Model file for the job. Use its own axes, mm. Face numbers are marked on the shaded views. A direction names the side the tool comes from. Coordinates: 2 decimals unless noted, no trailing zeros. Loops run counter-clockwise (first coordinate to the right, second up) from the corner with the lowest first, then second, coordinate; pieces in that order, holes last.
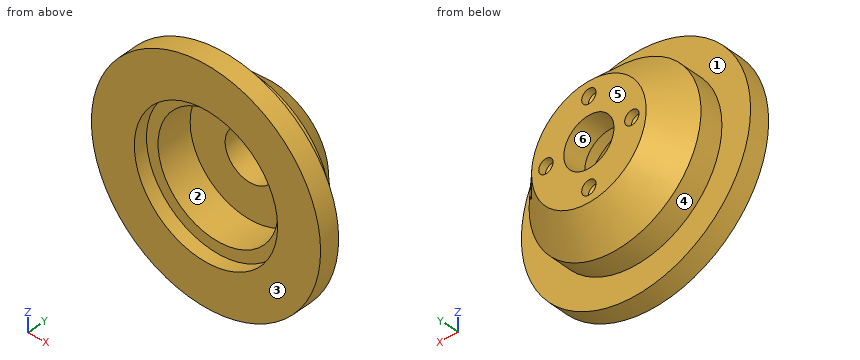
Autodesk Inventor part; units mm, degrees
ref_plane "Work Plane1" through (60, 0, 0) normal (1, 0, 0) x (0, 1, 0)
ref_plane "XZ Plane" through (0, 0, 0) normal (0, 1, 0) x (-1, 0, 0)
ref_plane "XY Plane" through (0, 0, 0) normal (0, 0, 1) x (1, 0, 0)
sketch "Sketch1" plane through (0, 0, 0) normal (0, 0, 1) x (1, 0, 0)
  line L0 (0, 0) -> (0, 66)
  line L1 (80, 0) -> (80, 13.8071)
  line L2 (-21.5975, 0) -> (0, 0)
  line L3 (46.9201, 0) -> (53.1744, 0)
  line L4 (80, 13.8071) -> (60, 13.8071)
  line L5 (60, 13.8071) -> (60, 33.8071)
  line L6 (36.9201, 33.8071) -> (30.3778, 33.8071)
  line L7 (0, 33.8071) -> (31.3863, 33.8071)
  line L8 (0, 33.8071) -> (0, 49.8071)
  line L9 (0, 49.8071) -> (35, 49.8071)
  line L10 (46.9201, 9.2823) -> (41.9201, 9.2823)
  line L11 (41.9201, 9.2823) -> (41.9201, 33.8071)
  line L12 (41.9201, 33.8071) -> (36.9201, 33.8071)
  line L13 (60, 33.8071) -> (60, 49.8071)
  line L14 (60, 49.8071) -> (35, 49.8071)
  line L15 (46.9201, 9.2823) -> (50, 9.2823)
  line L16 (50, 9.2823) -> (50, 0)
  line L17 (50, 0) -> (80, 0)
  dimension "d0" = 66
  dimension "d2" = 160
  dimension "d4" = 20
  dimension "d5" = 20
  dimension "d15" = 35
  dimension "d16" = 70
  dimension "d84" = 100
revolve "Revolution1" add sketch "Sketch1" angle 360 about axis through (0, 0, 0) along (0, 1, 0)
chamfer "Chamfer1" distance 20 angle 45 1 edges at (-60, 49.8071, 0)
ref_plane "Work Plane1" through (60, 0, 0) normal (1, 0, 0) x (0, 1, 0)
sketch "Sketch8" plane through (60, 0, 0) normal (1, 0, 0) x (0, 1, 0)
  circle A0 centre (51.2317, 0) radius 7.5
  point P0 (0, 0)
  dimension "d51" = 15
sketch "Sketch9" plane through (0, 0, 0) normal (0, 0, 1) x (1, 0, 0)
  line L0 (60.0797, 51.2451) -> (19.226, 26.5879)
  point P0 (0, 0)
sweep "Sweep2" cut profiles "Sketch8" path "Sketch9"
sketch "Sketch10" plane through (0, 49.8071, 0) normal (0, 1, 0) x (1, 0, 0)
  circle A0 centre (0, 0) radius 16
  dimension "d54" = 32
hole "Hole2" at (0, 49.8071, 0) direction (0, -1, 0) diameter 35 end through all
sketch "Sketch11" plane through (0, 49.8071, 0) normal (0, 1, 0) x (1, 0, 0)
  circle A0 centre (0, 0) radius 40
  circle A1 centre (0, -30) radius 5
  circle A2 centre (30, 0) radius 5
  circle A3 centre (0, 30) radius 5
  circle A4 centre (-30, 0) radius 5
  dimension "d64" = 80
  dimension "d65" = 10
  dimension "d66" = 30
  dimension "d67" = 360
hole "Hole3" at (0, 49.8071, -30) at (30, 49.8071, 0) at (0, 49.8071, 30) at (-30, 49.8071, 0) direction (0, -1, 0) diameter 10 depth 5 tip angle 118
thread "Thread5"
thread "Thread6"
thread "Thread7"
thread "Thread8"
equation "\"d60\" = Thickness"
equation "\"BendRadius\" = Thickness"
equation "\"BendReliefWidth\" = Thickness"
equation "\"BendReliefDepth\" = 0.5 * Thickness"
equation "\"CornerReliefSize\" = 4 * Thickness"
equation "\"MinimumRemnant\" = 2 * Thickness"
equation "\"TransitionRadius\" = BendRadius"
equation "\"JacobiRadiusSize\" = BendRadius"
equation "\"GapSize\" = Thickness"
properties material "Stainless Steel"
Q1. Flat gauge pins, fed straight in: P1, Ø6, axis at y = 30, z = -23, coming from the +X side; P2, Ø4, axis at x = 20, y = 43.5, coming from the -Z side; P3, Ø8, axis at x = 0, z = 30, coming from the +Y side. Where does each tip first touch, or does it go through?
Answers:
P1: stops at x = 56.57
P2: stops at z = -44.15
P3: stops at y = 44.21
Q2. Mould opens along Z. For the marked faces 4, 5 and 6 say: +Z half, -Z half, draft (parallel to the pull), parting line (faces both ways), or undercut.
Answers:
face 4: parting line
face 5: draft
face 6: undercut
Q3. Slice it at B-B (z = 62.5). List the corners of the cut face in (x, y), and give its area (3 significant figures).
Answers:
outline: (-49.94, 0) - (49.94, 0) - (49.94, 13.81) - (-49.94, 13.81) - close
area: 1,380 mm2
Q4. Drill centre lines: line 1 (X direction, y = 46.35, z = 0); line 2 (Z direction, x = 0, y = 44.75); line 3 (X direction, y = 22.5, z = 0). Where is each one in solid material? Low to high.
Answers:
line 1: x = -43.46 to -35, -25 to -17.5, 17.5 to 25, 35 to 39.49
line 2: z = -45.06 to -34.9, -25.1 to -17.5, 17.5 to 25.1, 34.9 to 45.06
line 3: x = -60 to -41.92, 41.92 to 60
Q5. Which spindle directions (+Z, -Z, +X, -X, +Y, -Y) get a long thin tool onto all of the face, cutting with end or side? Do the marked faces 1, 2 and 3. Say none if no direction does.
Answers:
face 1: +Y
face 2: -Y
face 3: +Z, -Z, +X, -X, -Y
Q6. Slice it at A-A (x = -64). List the corners of the cut face in (y, z).
Answers:
outline: (0, -48) - (13.81, -48) - (13.81, 48) - (0, 48) - close
